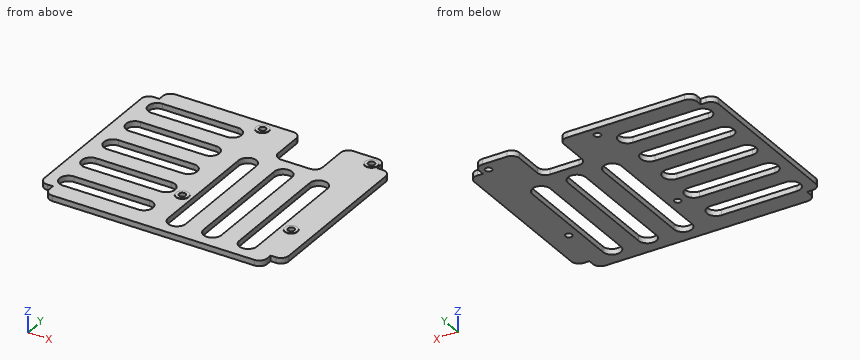
```python
from build123d import *

# Parameters (mm, degrees)
SKETCH_W                           = 110
SKETCH_H                           = 89
PAD_DEPTH                          = 2.5
SKETCH001_R                        = 2.9
PAD001_DEPTH                       = 0.2
SKETCH002_R                        = 1.5
POCKET_DEPTH                       = 2.701
SKETCH003_W                        = 20
SKETCH003_H                        = 20
POCKET001_DEPTH                    = 2.501
POCKET002_DEPTH                    = 285.543682
POCKET002_LINEARPATTERN_2_DEPTH    = 285.543682
LINEARPATTERN001_COUNT             = 2
LINEARPATTERN001_PITCH             = 16
POCKET003_DEPTH                    = 285.543682
POCKET003_LINEARPATTERN002_2_DEPTH = 285.543682
POCKET003_LINEARPATTERN002_3_DEPTH = 285.543682
LINEARPATTERN003_COUNT             = 3
LINEARPATTERN003_PITCH             = 16
FILLET_R                           = 3.5
SKETCH006_W                        = 6
SKETCH006_H                        = 6
POCKET004_DEPTH                    = 285.543682
FILLET001_R                        = 3.5


with BuildPart() as part:
    # Sketch → Pad (new body)
    with BuildSketch(Plane.XY):
        with Locations((55, 0)):
            Rectangle(SKETCH_W, SKETCH_H)
    extrude(amount=PAD_DEPTH)

    # Sketch001 (on Face6 of Pad) → Pad001 (join)
    with BuildSketch(Plane.XY.offset(2.5)):
        with Locations((100.5, 40)):
            Circle(SKETCH001_R)
        with Locations((100.5, -18)):
            Circle(SKETCH001_R)
        with Locations((51.5, 40)):
            Circle(SKETCH001_R)
        with Locations((51.5, -18)):
            Circle(SKETCH001_R)
    extrude(amount=PAD001_DEPTH)

    # Sketch002 (on Face13 of Pad001) → Pocket (cut, through all)
    with BuildSketch(Plane.XY.offset(2.7)):
        with Locations((51.5, 40)):
            Circle(SKETCH002_R)
        with Locations((100.5, 40)):
            Circle(SKETCH002_R)
        with Locations((51.5, -18)):
            Circle(SKETCH002_R)
        with Locations((100.5, -18)):
            Circle(SKETCH002_R)
    extrude(amount=-POCKET_DEPTH, mode=Mode.SUBTRACT)

    # Sketch003 → Pocket001 (cut, through all)
    with BuildSketch(Plane.XY.offset(2.5)):
        with Locations((76, 34.5)):
            Rectangle(SKETCH003_W, SKETCH003_H)
    extrude(amount=-POCKET001_DEPTH, mode=Mode.SUBTRACT)

    # Sketch004 (on Face5 of Pocket001) → Pocket002 (cut, through all)
    with BuildSketch(Plane.XY.offset(2.5)):
        with BuildLine():
            ThreePointArc((80, 15.5), (76, 19.5), (72, 15.5))
            Line((72, 15.5), (72, -35.5))
            ThreePointArc((72, -35.5), (76, -39.5), (80, -35.5))
            Line((80, 15.5), (80, -35.5))
        make_face()
    pocket002 = extrude(amount=-POCKET002_DEPTH, mode=Mode.SUBTRACT)

    # Sketch004 LinearPattern 2 → Pocket002 LinearPattern 2 (cut, through all)
    with BuildSketch(Plane(origin=(16, 0, 2.5), x_dir=(1, 0, 0), z_dir=(0, 0, 1))):
        with BuildLine():
            ThreePointArc((80, 15.5), (76, 19.5), (72, 15.5))
            Line((72, 15.5), (72, -35.5))
            ThreePointArc((72, -35.5), (76, -39.5), (80, -35.5))
            Line((80, 15.5), (80, -35.5))
        make_face()
    pocket002_linearpattern_2 = extrude(amount=-POCKET002_LINEARPATTERN_2_DEPTH, mode=Mode.SUBTRACT)

    # LinearPattern001: Pocket002, Pocket002 LinearPattern 2 ×2
    with Locations(*[(-i * LINEARPATTERN001_PITCH, 0, 0) for i in range(1, LINEARPATTERN001_COUNT)]):
        add(pocket002, mode=Mode.SUBTRACT)
        add(pocket002_linearpattern_2, mode=Mode.SUBTRACT)

    # Sketch005 (on Face5 of MultiTransform) → Pocket003 (cut, through all)
    with BuildSketch(Plane.XY.offset(2.5)):
        with BuildLine():
            ThreePointArc((9, 4), (5, 0), (9, -4))
            Line((9, -4), (43, -4))
            ThreePointArc((43, -4), (47, 0), (43, 4))
            Line((9, 4), (43, 4))
        make_face()
    pocket003 = extrude(amount=-POCKET003_DEPTH, mode=Mode.SUBTRACT)

    # Sketch005 LinearPattern002 2 → Pocket003 LinearPattern002 2 (cut, through all)
    with BuildSketch(Plane(origin=(0, 16, 2.5), x_dir=(1, 0, 0), z_dir=(0, 0, 1))):
        with BuildLine():
            ThreePointArc((9, 4), (5, 0), (9, -4))
            Line((9, -4), (43, -4))
            ThreePointArc((43, -4), (47, 0), (43, 4))
            Line((9, 4), (43, 4))
        make_face()
    pocket003_linearpattern002_2 = extrude(amount=-POCKET003_LINEARPATTERN002_2_DEPTH, mode=Mode.SUBTRACT)

    # Sketch005 LinearPattern002 3 → Pocket003 LinearPattern002 3 (cut, through all)
    with BuildSketch(Plane(origin=(0, 32, 2.5), x_dir=(1, 0, 0), z_dir=(0, 0, 1))):
        with BuildLine():
            ThreePointArc((9, 4), (5, 0), (9, -4))
            Line((9, -4), (43, -4))
            ThreePointArc((43, -4), (47, 0), (43, 4))
            Line((9, 4), (43, 4))
        make_face()
    pocket003_linearpattern002_3 = extrude(amount=-POCKET003_LINEARPATTERN002_3_DEPTH, mode=Mode.SUBTRACT)

    # LinearPattern003: Pocket003, Pocket003 LinearPattern002 2, Pocket003 LinearPattern002 3 ×3
    with Locations(*[(0, -i * LINEARPATTERN003_PITCH, 0) for i in range(1, LINEARPATTERN003_COUNT)]):
        add(pocket003, mode=Mode.SUBTRACT)
        add(pocket003_linearpattern002_2, mode=Mode.SUBTRACT)
        add(pocket003_linearpattern002_3, mode=Mode.SUBTRACT)

    # Fillet
    fillet_edges = [part.edges().sort_by_distance(p)[0] for p in [
        (110, 44.5, 1.25),
        (66, 44.5, 1.25),
        (66, 24.5, 1.25),
        (110, -44.5, 1.25),
        (86, 44.5, 1.25),
        (86, 24.5, 1.25),
        (0, 44.5, 1.25),
        (0, -44.5, 1.25),
    ]]
    fillet(fillet_edges, radius=FILLET_R)

    # Sketch006 (on Face5 of Fillet) → Pocket004 (cut, through all)
    with BuildSketch(Plane.XY.offset(2.5)):
        with Locations((107, 41.5)):
            Rectangle(SKETCH006_W, SKETCH006_H)
        with Locations((3, 41.5)):
            Rectangle(SKETCH006_W, SKETCH006_H)
    pocket004 = extrude(amount=-POCKET004_DEPTH, mode=Mode.SUBTRACT)

    # Mirrored: Pocket004 across XZ
    add(pocket004.mirror(Plane.XZ), mode=Mode.SUBTRACT)

    # Fillet001
    fillet001_edges = [part.edges().sort_by_distance(p)[0] for p in [
        (110, -38.5, 1.25),
        (104, -44.5, 1.25),
        (110, 38.5, 1.25),
        (104, 44.5, 1.25),
        (6, 44.5, 1.25),
        (0, 38.5, 1.25),
        (0, -38.5, 1.25),
        (6, -44.5, 1.25),
    ]]
    fillet(fillet001_edges, radius=FILLET001_R)


solid = part.part
```
Geometry: final body of the model. Coordinates: model frame, mm. Round coordinates to 2 decimals unless told otherwise and drop trailing zeros. Order: outer loops, then holes, each group sorted by start corner. A loop starts at its lowest first (then second) coordinate and runs counter-clockwise, first axis right, second up. Notation, with made-up numbers: (32.5, 26) -> (80.5, 26) arc R20 cw to (80.5, 65) -> close; hole circle Ø3 at (77.25, 60.5). An arc over 180 degrees is marked (long way). Use CSV: the item, a comma, the result in double quotes. Start each with the question number.
1) Section C-C (x = 92). Return the cut outline in (y, z).
2) Section A-A (y = -24). Return the cut outline in (x, z).
3) First-contact query: pin 1 Ø0.8 at (x, z) = (105, 1) entering from -Y; pin 2 Ø1.8 at (x, y) = (100.5, 40) entering from +Z; pin 3 Ø5 at (x, y) = (31.5, -21) entering from +Z. Flat tips, straight axial feed; report the tip coordinate or a pass-through.
4) Material intervals for line 1 along X through (y, z) = (-32, 0.65); line 2 along Y through (x, z) = (51.5, 0.95); line 3 along X through (y, z) = (-11.5, 1), sorted ascending. Write a range as from..to.
5) Section D-D (x = 76). Return the cut outline in (y, z), and give its area (3 significant figures).
6) Section B-B (y = 32). Return the cut outline in (x, z), and give its area (3 significant figures).
Returned:
1,outline,"(-44.5, 0) -> (-39.5, 0) -> (-39.5, 2.5) -> (-44.5, 2.5) -> close; (19.5, 0) -> (44.5, 0) -> (44.5, 2.5) -> (19.5, 2.5) -> close"
2,outline,"(0, 0) -> (56, 0) -> (56, 2.5) -> (0, 2.5) -> close; (64, 0) -> (72, 0) -> (72, 2.5) -> (64, 2.5) -> close; (80, 0) -> (88, 0) -> (88, 2.5) -> (80, 2.5) -> close; (96, 0) -> (110, 0) -> (110, 2.5) -> (96, 2.5) -> close"
3,pin 1,"stops at y = -38.5"
3,pin 2,"passes through"
3,pin 3,"stops at z = 2.5"
4,line 1,"x = 0..5, 47..56, 64..72, 80..88, 96..110"
4,line 2,"y = -44.5..-19.5, -16.5..38.5, 41.5..44.5"
4,line 3,"x = 0..56, 64..72, 80..88, 96..110"
5,outline,"(-44.5, 0) -> (-39.5, 0) -> (-39.5, 2.5) -> (-44.5, 2.5) -> close; (19.5, 0) -> (24.5, 0) -> (24.5, 2.5) -> (19.5, 2.5) -> close"
5,area,"25.0 mm²"
6,outline,"(0, 0) -> (5, 0) -> (5, 2.5) -> (0, 2.5) -> close; (47, 0) -> (66, 0) -> (66, 2.5) -> (47, 2.5) -> close; (86, 0) -> (110, 0) -> (110, 2.5) -> (86, 2.5) -> close"
6,area,"120 mm²"
